Geometry check sheet. Reference: the model listing, model coordinates, mm. A direction names the side the tool comes from. Coordinates: 2 decimals unless noted, no trailing zeros. Loops run counter-clockwise (first coordinate to the right, second up) from the corner with the lowest first, then second, coordinate; pieces in that order, holes last.
from build123d import *

# Parameters (mm, degrees)
F1_DEPTH      = 152.4
F1_DEPTH_BACK = 152.4
F2_R          = 19.05
F3_DEPTH      = 76.2


with BuildPart() as f1:
    # F0 (on Top) → F1 (new body, two sides)
    with BuildSketch(Plane.XY) as f1_sk:
        Polygon((-31.75, 50.8), (31.75, 50.8), (31.75, -50.8), (38.1, -50.8), (38.1, 57.15), (-38.1, 57.15), (-38.1, -50.8), (-31.75, -50.8), align=None)
    extrude(amount=F1_DEPTH)
    extrude(f1_sk.sketch, amount=-F1_DEPTH_BACK)

    # F2 (on face) → F3 (join)
    with BuildSketch(Plane(origin=(-38.1, 0, 0), x_dir=(0, -1, 0), z_dir=(-1, 0, 0))):
        with Locations((0, 101.6)):
            Circle(F2_R)
    extrude(amount=-F3_DEPTH)

    # F4: F1 across plane


with BuildPart() as f1_1:
    add(f1.part)
    add(f1.part.mirror(Plane.XY))


solid = f1_1.part
(1) Sectioned sample at D-D on z = -15.5. Record the cut outline in (x, y).
Findings:
outline: (-38.1, -50.8) - (-31.75, -50.8) - (-31.75, 50.8) - (31.75, 50.8) - (31.75, -50.8) - (38.1, -50.8) - (38.1, 57.15) - (-38.1, 57.15) - close
(2) Draft check along Z on faces 4 (the cylindrical face through (-0.445, 2.48, 120.488)), 5 (the flat face through (-34, 19, -152.4)), 6 (the flat face through (-34, 19, 152.4)). Enter one of: +Z half, -Z half, draft (parallel to the pull), parting line (faces both ways), or undercut.
Findings:
face 4: undercut
face 5: -Z half
face 6: +Z half
(3) Scan lines: L1, parallel to X at y = -8, z = 136; L2, parallel to Y at x = -23, z = 124.5. Record each from-to range of solid material in increasing order.
Findings:
L1: x = -38.1 to -31.75, 31.75 to 38.1
L2: y = 50.8 to 57.15
(4) Sectioned sample at A-A on z = 101.6. Record the cut outline in (x, y), and give its area (3 significant figures).
Findings:
outline: (-38.1, -50.8) - (-31.75, -50.8) - (-31.75, -19.05) - (31.75, -19.05) - (31.75, -50.8) - (38.1, -50.8) - (38.1, 57.15) - (-38.1, 57.15) - close; hole (-31.75, 19.05) - (31.75, 19.05) - (31.75, 50.8) - (-31.75, 50.8) - close
area: 4,190 mm2
(5) Sectioned sample at C-C on y = 0. Record the cut outline in (x, z).
Findings:
outline: (-38.1, -152.4) - (-31.75, -152.4) - (-31.75, -120.65) - (31.75, -120.65) - (31.75, -152.4) - (38.1, -152.4) - (38.1, 152.4) - (31.75, 152.4) - (31.75, 120.65) - (-31.75, 120.65) - (-31.75, 152.4) - (-38.1, 152.4) - close; hole (-31.75, -82.55) - (31.75, -82.55) - (31.75, 82.55) - (-31.75, 82.55) - close
(6) Gauge pin test, flat ends, axial feed: pin 1 Ø1.5 at (x, z) = (-16, -79) entering from -Y; pin 2 Ø10 at (x, y) = (-21.5, -15.5) entering from +Z. Record the tip position at first contact, or that the pin passes through.
Findings:
pin 1: stops at y = 50.8
pin 2: stops at z = 117.5
(7) Sectioned sample at B-B on x = 17.5. Record the cut outline in (y, z).
Findings:
outline: circle Ø38.1 at (0, -101.6); circle Ø38.1 at (0, 101.6); (50.8, -152.4) - (57.15, -152.4) - (57.15, 152.4) - (50.8, 152.4) - close
(8) Access from +Z, -Z, +X, -X, +Y, -Y to the whole of each face (thin tool, end or side, straight path). Record for faces 1 (the cylindrical face through (-0.445, 2.48, -120.488)), 2 (the flat face through (-35, -50.8, 2)), 3 (the flat face through (0, 50.8, 2)).
Findings:
face 1: none
face 2: +Z, -Z, +X, -X, -Y
face 3: +Z, -Z
